Verification items for the finished model (mm, model axes). Face numbers are marked on the shaded views. A direction names the side the tool comes from. Give positions to 0.01 mm unless a question says otherwise; leave off trailing zeros. Order: outer loops, then holes, each group sorted by start corner. A loop starts at its lowest first (then second) coordinate and runs counter-clockwise, first axis right, second up. Notation, with made-up numbers: (32, 84) - (69, 84) arc R25 cw to (69, 111) - close; hole circle Ø9 at (9, 61.25). An arc over 180 degrees is marked (long way). Answer as a JSON object with one key per item and string values. Group by question number.
(1) Mould release check, pull along X, two halves, no side actions. Record for the marked faces 5, 6 and 7: +X half, -X half, draft (parallel to the pull), parting line (faces both ways), or undercut.
(2) Thickness scan on line 1 (Z direction, x = 7.5, y = 2.5); line 2 (X direction, y = -0.75, z = -5); line 3 (Y direction, x = -14, z = 0.35). Record the ranges inside material, lowest first.
(3) Section check B-B (x = -14). Record the boundary of the cut face in (y, z), then the cut area to 3 significant figures.
(4) Depth check by flat-ended pin: pin 1 Ø3.5 at (x, y) = (-3, -2.5) entering from -Z; pin 2 Ø2 at (y, z) = (0, -17) entering from +X; pin 3 Ø2 at (y, z) = (4.5, -10.5) entering from -X; pin 4 Ø1.1 at (x, z) = (1.5, 2.5) entering from -Y. Enter the tip coordinate at first touch or a pass-through.
(5) Section check D-D (y = -3.25). Record the boundary of the cut face in (x, z), then the cut area to 3 significant figures.
(6) Section check A-A (z = -1.5). Record the boundary of the cut face in (x, y), then the cut area to 3 significant figures.
(7) Section check C-C (y = 0). Count the separate pieces of the cut face and the enclosed holes in it, then the cut area to 3 significant figures.
(8) Access from +Z, -Z, +X, -X, +Y, -Y to the whole of each face (thin tool, end or side, straight path). Record for the marked faces 1, 2, 3 and 4.
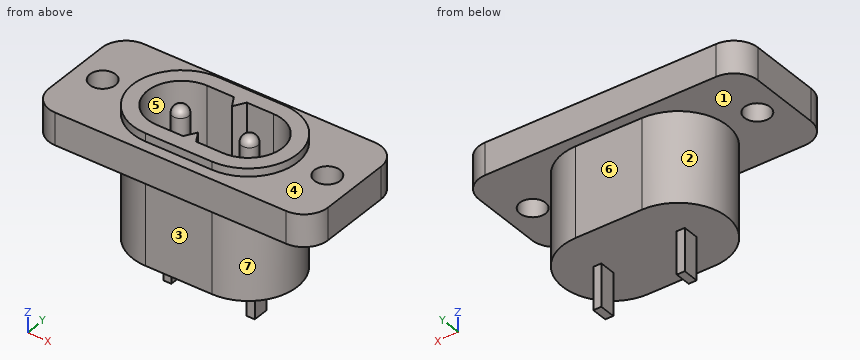
```python
from build123d import *

# Parameters (mm, degrees)
SKETCH1_R                = 1.6
BOSS_EXTRUDE1_DEPTH      = 2
BOSS_EXTRUDE2_DEPTH      = 1
BOSS_EXTRUDE2_DEPTH_BACK = 15.2
BOSS_EXTRUDE3_START      = -9.8
BOSS_EXTRUDE3_DEPTH      = 1
BOSS_EXTRUDE4_START      = 5.2
BOSS_EXTRUDE4_DEPTH      = 0.5
BOSS_EXTRUDE6_DEPTH      = 1
SKETCH6_R                = 1
BOSS_EXTRUDE7_DEPTH      = 8.8
FILLET1_R                = 1


with BuildPart() as part:
    # Sketch1 → Boss-Extrude1 (new, symmetric)
    with BuildSketch(Plane.XY):
        with BuildLine():
            Line((-14.4, 7.45), (14.4, 7.45))
            ThreePointArc((14.4, 7.45), (16.521320344, 6.571320344), (17.4, 4.45))
            Line((17.4, 4.45), (17.4, -4.45))
            ThreePointArc((17.4, -4.45), (16.521320344, -6.571320344), (14.4, -7.45))
            Line((14.4, -7.45), (-14.4, -7.45))
            ThreePointArc((-14.4, -7.45), (-16.521320344, -6.571320344), (-17.4, -4.45))
            Line((-17.4, -4.45), (-17.4, 4.45))
            ThreePointArc((-17.4, 4.45), (-16.521320344, 6.571320344), (-14.4, 7.45))
        make_face()
        with Locations((14, 0)):
            Circle(SKETCH1_R, mode=Mode.SUBTRACT)
        with Locations(Location((-14, 0, 0), (0, 0, 180))):
            Circle(SKETCH1_R, mode=Mode.SUBTRACT)
        with BuildLine():
            Line((-4.15, 4.25), (-0.808290377, 4.25))
            Line((-0.808290377, 4.25), (0, 2.85))
            Line((0, 2.85), (0.808290377, 4.25))
            Line((0.808290377, 4.25), (4.15, 4.25))
            ThreePointArc((4.15, 4.25), (8.4, 0), (4.15, -4.25))
            Line((4.15, -4.25), (0.808290377, -4.25))
            Line((0.808290377, -4.25), (0, -2.85))
            Line((0, -2.85), (-0.808290377, -4.25))
            Line((-0.808290377, -4.25), (-4.15, -4.25))
            ThreePointArc((-4.15, -4.25), (-8.4, 0), (-4.15, 4.25))
        make_face(mode=Mode.SUBTRACT)
    extrude(amount=BOSS_EXTRUDE1_DEPTH, both=True)

    # Sketch2 → Boss-Extrude2 (add, two sides: drawn at the far end of the back side and taken through both)
    with BuildSketch(Plane.XY.offset(2).offset(-BOSS_EXTRUDE2_DEPTH_BACK)):
        with BuildLine():
            Line((-4.15, 6.1), (4.15, 6.1))
            ThreePointArc((4.15, 6.1), (10.25, 0), (4.15, -6.1))
            Line((4.15, -6.1), (-4.15, -6.1))
            ThreePointArc((-4.15, -6.1), (-10.25, 0), (-4.15, 6.1))
        make_face()
        with BuildLine():
            Line((0.808290377, 4.25), (0, 2.85))
            Line((0, 2.85), (-0.808290377, 4.25))
            Line((-0.808290377, 4.25), (-4.15, 4.25))
            ThreePointArc((-4.15, 4.25), (-8.4, 0), (-4.15, -4.25))
            Line((-4.15, -4.25), (-0.808290377, -4.25))
            Line((-0.808290377, -4.25), (0, -2.85))
            Line((0, -2.85), (0.808290377, -4.25))
            Line((0.808290377, -4.25), (4.15, -4.25))
            ThreePointArc((4.15, -4.25), (8.4, 0), (4.15, 4.25))
            Line((4.15, 4.25), (0.808290377, 4.25))
        make_face(mode=Mode.SUBTRACT)
    extrude(amount=BOSS_EXTRUDE2_DEPTH + BOSS_EXTRUDE2_DEPTH_BACK)

    # Sketch3 → Boss-Extrude3 (add)
    with BuildSketch(Plane.XY.offset(3).offset(BOSS_EXTRUDE3_START)):
        with BuildLine():
            Line((0.808290377, 4.25), (0, 2.85))
            Line((0, 2.85), (-0.808290377, 4.25))
            Line((-0.808290377, 4.25), (-4.15, 4.25))
            ThreePointArc((-4.15, 4.25), (-8.4, 0), (-4.15, -4.25))
            Line((-4.15, -4.25), (-0.808290377, -4.25))
            Line((-0.808290377, -4.25), (0, -2.85))
            Line((0, -2.85), (0.808290377, -4.25))
            Line((0.808290377, -4.25), (4.15, -4.25))
            ThreePointArc((4.15, -4.25), (8.4, 0), (4.15, 4.25))
            Line((4.15, 4.25), (0.808290377, 4.25))
        make_face()
    extrude(amount=BOSS_EXTRUDE3_DEPTH)



with BuildPart() as body_2:
    # Sketch4 → Boss-Extrude4 (new, symmetric)
    with BuildSketch(Plane(origin=(0, 0, 0), x_dir=(0, 0, -1), z_dir=(1, 0, 0)).offset(BOSS_EXTRUDE4_START)):
        Polygon((13.2, 1), (15.8, 1), (18.5, 1), (18.5, -1), (13.8, -1), (13.2, -1), align=None)
    boss_extrude4 = extrude(amount=BOSS_EXTRUDE4_DEPTH, both=True)


with BuildPart() as part_1:
    add(part.part)

    add(body_2.part)  # Boss-Extrude6 merges body 2
    # Sketch5 → Boss-Extrude6 (add)
    with BuildSketch(Plane(origin=(0, 0, -13.2), x_dir=(-1, 0, 0), z_dir=(0, 0, -1))):
        with BuildLine():
            Line((4.15, 6.1), (-4.15, 6.1))
            ThreePointArc((-4.15, 6.1), (-10.25, 0), (-4.15, -6.1))
            Line((-4.15, -6.1), (4.15, -6.1))
            ThreePointArc((4.15, -6.1), (10.25, 0), (4.15, 6.1))
        make_face()
    extrude(amount=-BOSS_EXTRUDE6_DEPTH)

    # Mirror2: Boss-Extrude4 across plane
    add(boss_extrude4.mirror(Plane(origin=(0, 0, 0), x_dir=(0, 0, 1), z_dir=(1, 0, 0))))

    # Sketch6 → Boss-Extrude7 (add)
    with BuildSketch(Plane.XY.offset(-5.8)):
        with Locations((-4.3, 0)):
            Circle(SKETCH6_R)
        with Locations(Location((4.3, 0, 0), (0, 0, 180))):
            Circle(SKETCH6_R)
    extrude(amount=BOSS_EXTRUDE7_DEPTH)

    # Fillet1
    fillet1_edges = [part_1.edges().sort_by_distance(p)[0] for p in [
        (-5.3, 0, 3),
        (5.3, 0, 3),
    ]]
    fillet(fillet1_edges, radius=FILLET1_R)


solid = part_1.part
```
Solutions:
{
 "1": {"face 5": "undercut", "face 6": "draft", "face 7": "+X half"},
 "2": {"line 1": "z = -13.2 to -12.2, -6.8 to -5.8", "line 2": "x = -10.2 to -8.33, -4.96 to -3.64, 3.64 to 4.96, 8.33 to 10.2", "line 3": "y = -7.45 to -1.6, 1.6 to 7.45"},
 "3": {"outline": "(-7.45, -2) - (-1.6, -2) - (-1.6, 2) - (-7.45, 2) - close; (1.6, -2) - (7.45, -2) - (7.45, 2) - (1.6, 2) - close", "area": "46.8 mm2"},
 "4": {"pin 1": "stops at z = -13.2", "pin 2": "stops at x = 5.7", "pin 3": "stops at x = -9.15", "pin 4": "stops at y = -7.45"},
 "5": {"outline": "(-17.4, -2) - (-9.31, -2) - (-9.31, -13.2) - (9.31, -13.2) - (9.31, -2) - (17.4, -2) - (17.4, 2) - (9.31, 2) - (9.31, 3) - (6.89, 3) - (6.89, -5.8) - (0.23, -5.8) - (0.23, 3) - (-0.23, 3) - (-0.23, -5.8) - (-6.89, -5.8) - (-6.89, 3) - (-9.31, 3) - (-9.31, 2) - (-17.4, 2) - close; hole (-6.89, -12.2) - (-0.23, -12.2) - (-0.23, -6.8) - (-6.89, -6.8) - close; hole (0.23, -12.2) - (6.89, -12.2) - (6.89, -6.8) - (0.23, -6.8) - close", "area": "177 mm2"},
 "6": {"outline": "(-17.4, -4.45) arc R3 ccw to (-14.4, -7.45) - (14.4, -7.45) arc R3 ccw to (17.4, -4.45) - (17.4, 4.45) arc R3 ccw to (14.4, 7.45) - (-14.4, 7.45) arc R3 ccw to (-17.4, 4.45) - close; circle Ø2 at (-4.3, 0); circle Ø2 at (4.3, 0); hole circle Ø3.2 at (-14, 0); hole (-4.15, -4.25) - (-0.81, -4.25) - (0, -2.85) - (0.81, -4.25) - (4.15, -4.25) arc R4.25 ccw to (4.15, 4.25) - (0.81, 4.25) - (0, 2.85) - (-0.81, 4.25) - (-4.15, 4.25) arc R4.25 ccw to start; hole circle Ø3.2 at (14, 0)", "area": "376 mm2"},
 "7": {"separate pieces": "3", "enclosed holes": "1", "area": "170 mm2"},
 "8": {"face 1": "-Z", "face 2": "-Z, -X", "face 3": "-Z, +X, -X, -Y", "face 4": "+Z"}
}
